Geometry: final body of the model. Coordinates: model frame, mm. Give positions to 0.01 mm unless a question says otherwise; leave off trailing zeros. Write each loop counter-clockwise with the first axis right and the second up, starting at its lowest first coordinate (ties: lowest second). Pieces come first, ordered by that corner, then holes.
from build123d import *

# Parameters (mm, degrees)
F0_W     = 30
F0_H     = 5
F0_R     = 1.5
F1_DEPTH = 2.5


with BuildPart() as f1:
    # F0 (on Front) → F1 (new body, symmetric)
    with BuildSketch(Plane.XZ):
        with Locations((15, 2.5)):
            Rectangle(F0_W, F0_H)
        with Locations((3, 2.5)):
            Circle(F0_R, mode=Mode.SUBTRACT)
        with Locations((27, 2.5)):
            Circle(F0_R, mode=Mode.SUBTRACT)
    extrude(amount=F1_DEPTH, both=True)


solid = f1.part
Q1. Section B-B on x = 3. Output: boundary loops of the cut face in (y, z).
Filled sheet:
outline: (-2.5, 0) - (2.5, 0) - (2.5, 1) - (-2.5, 1) - close; (-2.5, 4) - (2.5, 4) - (2.5, 5) - (-2.5, 5) - close
Q2. Section C-C on y = 2.15. Output: boundary loops of the cut face in (x, z).
Filled sheet:
outline: (0, 0) - (30, 0) - (30, 5) - (0, 5) - close; hole circle Ø3 at (3, 2.5); hole circle Ø3 at (27, 2.5)
Q3. Section A-A on z = 2.5. Output: boundary loops of the cut face in (x, y).
Filled sheet:
outline: (0, -2.5) - (1.5, -2.5) - (1.5, 2.5) - (0, 2.5) - close; (4.5, -2.5) - (25.5, -2.5) - (25.5, 2.5) - (4.5, 2.5) - close; (28.5, -2.5) - (30, -2.5) - (30, 2.5) - (28.5, 2.5) - close
Q4. Pin query (flat end, axial travel): P1, Ø2.5, axis at x = 3, z = 2.5, coming from the +Y side. Return the tip coordinate at first contact, or that it passes through.
Filled sheet:
P1: passes through
Q5. Pull-direction query (Z, two-part tool) for faces 1 (the flat face through (15, 0, 0)), 2 (the cylindrical face through (25.5, 0.04, 2.57)), 3 (the flat face through (0, 0, 2)); classes: released by +Z, released by -Z, zero draft, split by the parting line, or undercut.
Filled sheet:
face 1: released by -Z
face 2: undercut
face 3: zero draft
Q6. Ray query, line 1 along Z through (x, y) = (3, 1.25); line 2 along X through (y, z) = (-1.3, 2.45); line 3 along X through (y, z) = (1.15, 1.75). Return the intervals inside material, ascending.
Filled sheet:
line 1: z = 0 to 1, 4 to 5
line 2: x = 0 to 1.5, 4.5 to 25.5, 28.5 to 30
line 3: x = 0 to 1.7, 4.3 to 25.7, 28.3 to 30
Q7. Section D-D on x = 27.5. Output: boundary loops of the cut face in (y, z), plus the area to 3 significant figures.
Filled sheet:
outline: (-2.5, 0) - (2.5, 0) - (2.5, 1.09) - (-2.5, 1.09) - close; (-2.5, 3.91) - (2.5, 3.91) - (2.5, 5) - (-2.5, 5) - close
area: 10.9 mm2
